Autodesk Inventor part; units mm, degrees
ref_plane "YZ Plane" through (0, 0, 0) normal (1, 0, 0) x (0, 1, 0)
ref_plane "XZ Plane" through (0, 0, 0) normal (0, 1, 0) x (-1, 0, 0)
ref_plane "XY Plane" through (0, 0, 0) normal (0, 0, 1) x (1, 0, 0)
sketch "Esquisse1" plane through (0, 0, 0) normal (0, 0, 1) x (1, 0, 0)
  line L0 (0, 0) -> (5, 0)
  line L1 (5, 0) -> (5, 90)
  line L2 (5, 90) -> (0, 90)
  line L3 (0, 90) -> (0, 0)
  dimension "d0" = 10
  dimension "d3" = 180
revolve "Révolution1" add sketch "Esquisse1" angle 360 about axis through (0, 90, 0) along (0, -1, 0)
sketch "Esquisse2" plane through (0, 90, 0) normal (0, 1, 0) x (1, 0, 0)
  circle A0 centre (0, 0) radius 5
hole "Perçage1" at (0, 90, 0) direction (0, -1, 0) diameter 3.242 depth 20 tip angle 118
mirror "Mise en miroir1" about plane through (0, 0, 0) normal (0, 1, 0)
properties part number "barre" material "Aluminium 6061"
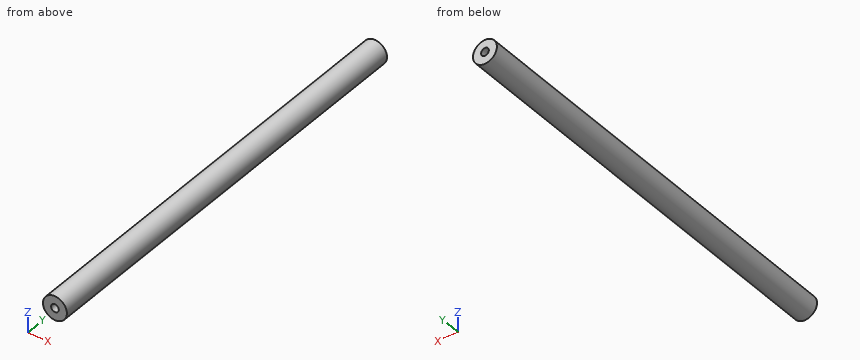
Verification items for the finished model (mm, model axes). Round coordinates to 2 decimals unless told otherwise and drop trailing zeros. Loops run counter-clockwise (first coordinate to the right, second up) from the corner with the lowest first, then second, coordinate; pieces in that order, holes last. Notation, with made-up numbers: M 33,-25.75 L 46,-25.75 A25 cw 46,-1.75 Z; hole C 55,-24 d10. An arc over 180 degrees is marked long. Write each question's results on one line, items separated by ' | '.
1) Section check A-A on y = 0. Record the boundary of the cut face in (x, z).
Checks:
outline: C 0,0 d10
2) Scan lines: L1, parallel to Z at x = 0, y = -75.5; L2, parallel to Z at x = -0.5, y = 60.5; L3, parallel to X at y = 37.5, z = -0.25. Record each from-to range of solid material in increasing order. Write a range as from..to.
Checks:
L1: z = -5..-1.62, 1.62..5 | L2: z = -4.97..4.97 | L3: x = -4.99..4.99
3) Gauge pin test, flat ends, axial feed: P1, Ø4, axis at x = -3.5, y = 47, coming from the +Z side; P2, Ø2.5, axis at x = 0, z = 0, coming from the -Y side; P3, Ø1.5, axis at x = -3, y = 9, coming from the +Z side. Record the tip position at first contact, or that the pin passes through.
Checks:
P1: stops at z = 4.77 | P2: stops at y = -69.78 | P3: stops at z = 4.47
4) Section check B-B on x = 3.5. Record the boundary of the cut face in (y, z), then the cut area to 3 significant figures.
Checks:
outline: M -90,-3.57 L 90,-3.57 L 90,3.57 L -90,3.57 Z | area: 1,290 mm2
